Read the model definition and answer for the solid it produces. Units are mm, in the model's axes. A direction names the side the tool comes from. Coordinates: 2 decimals unless noted, no trailing zeros. Loops run counter-clockwise (first coordinate to the right, second up) from the corner with the lowest first, then second, coordinate; pieces in that order, holes last.
from build123d import *

# Parameters (mm, degrees)
SKETCH1_R           = 53.5
BOSS_EXTRUDE1_DEPTH = 2
SKETCH2_R           = 2.7
BOSS_EXTRUDE2_DEPTH = 2
SKETCH3_R           = 3.55
CUT_EXTRUDE1_DEPTH  = 2
SKETCH7_R           = 53.5
SKETCH7_R_2         = 52
BOSS_EXTRUDE3_DEPTH = 10
SKETCH8_W           = 56.651812746
SKETCH8_H           = 12.7
CUT_EXTRUDE4_DEPTH  = 10
SKETCH13_R          = 52.5
SKETCH13_R_2        = 3.55
BOSS_EXTRUDE4_DEPTH = 2
SKETCH12_R          = 2.75
CUT_EXTRUDE6_DEPTH  = 3
SKETCH16_R          = 1.5
CUT_EXTRUDE8_DEPTH  = 2


with BuildPart() as part:
    # Sketch1 → Boss-Extrude1 (new body)
    with BuildSketch(Plane(origin=(0, 0, 0), x_dir=(1, 0, 0), z_dir=(0, 1, 0))):
        Circle(SKETCH1_R)
    extrude(amount=BOSS_EXTRUDE1_DEPTH)

    # Sketch2 → Boss-Extrude2 (add)
    with BuildSketch(Plane(origin=(0, 2, 0), x_dir=(1, 0, 0), z_dir=(0, 1, 0))):
        with Locations((0, -44.45)):
            Circle(SKETCH2_R)
        with Locations((0, 44.45)):
            Circle(SKETCH2_R)
    extrude(amount=BOSS_EXTRUDE2_DEPTH)

    # Sketch3 → Cut-Extrude1 (cut)
    with BuildSketch(Plane(origin=(0, 2, 0), x_dir=(1, 0, 0), z_dir=(0, 1, 0))):
        Circle(SKETCH3_R)
    extrude(amount=-CUT_EXTRUDE1_DEPTH, mode=Mode.SUBTRACT)

    # Sketch7 → Boss-Extrude3 (add)
    with BuildSketch(Plane(origin=(0, 2, 0), x_dir=(1, 0, 0), z_dir=(0, 1, 0))):
        Circle(SKETCH7_R)
        Circle(SKETCH7_R_2, mode=Mode.SUBTRACT)
    extrude(amount=BOSS_EXTRUDE3_DEPTH)

    # Sketch8 → Cut-Extrude4 (cut)
    with BuildSketch(Plane(origin=(0, 2, 0), x_dir=(1, 0, 0), z_dir=(0, 1, 0))):
        with Locations((-28.325906373, 0)):
            Rectangle(SKETCH8_W, SKETCH8_H)
    extrude(amount=CUT_EXTRUDE4_DEPTH, mode=Mode.SUBTRACT)

    # Sketch13 → Boss-Extrude4 (add)
    with BuildSketch(Plane.XZ):
        Circle(SKETCH13_R)
        Circle(SKETCH13_R_2, mode=Mode.SUBTRACT)
    extrude(amount=BOSS_EXTRUDE4_DEPTH)

    # Sketch12 → Cut-Extrude6 (cut)
    with BuildSketch(Plane(origin=(0, 2, 0), x_dir=(1, 0, 0), z_dir=(0, 1, 0))):
        with Locations((11.16900504, 10.012658309)):
            Circle(SKETCH12_R)
        with Locations((-0.61610798, -14.987341691)):
            Circle(SKETCH12_R)
        with Locations((-13.568010506, 6.396021491)):
            Circle(SKETCH12_R)
    extrude(amount=-CUT_EXTRUDE6_DEPTH, mode=Mode.SUBTRACT)

    # Sketch16 → Cut-Extrude8 (cut, through all)
    with BuildSketch(Plane(origin=(0, -1, 0), x_dir=(1, 0, 0), z_dir=(0, 1, 0))):
        with Locations((11.16900504, 10.012658309)):
            Circle(SKETCH16_R)
        with Locations((-0.61610798, -14.987341691)):
            Circle(SKETCH16_R)
        with Locations((-13.568010506, 6.396021491)):
            Circle(SKETCH16_R)
    extrude(amount=-CUT_EXTRUDE8_DEPTH, mode=Mode.SUBTRACT)


solid = part.part
Q1. Flat-ended cylindrical pins translate along their axes: pin 1 Ø4.5 at (x, z) = (-1, -45.5) entering from +Y; pin 2 Ø9 at (x, z) = (-13.57, -6.4) entering from +Y; pin 3 Ø3.5 at (x, z) = (11.17, -10.01) entering from +Y; pin 4 Ø6.5 at (x, z) = (0, 0) entering from -Y. Find the tip coordinate at first contact, or state that the pin passes through.
Findings below:
pin 1: stops at y = 4
pin 2: stops at y = 2
pin 3: stops at y = -1
pin 4: passes through
Q2. Which of the six approach directions +Z, -Z, +X, -X, +Y, -Y give full straight-line access (tool end or side, diameter ignored) to faces 1 (the face through (35.4, 0, 39.4)), 2 (the face through (49.42, 5.92, 20.49)), 3 (the face through (1.246, 2.986, -42.055))?
Findings below:
face 1: -Y
face 2: +Y, -Y
face 3: +Y
Q3. Straight lines are drawn through the part: probe 1 along Y at (x, z) = (-44, -24); probe 2 along Z at (x, y) = (0, 1.25); probe 3 along Z at (x, y) = (19, 11.25). For each, find the intervals that lie inside material, in ascending order.
Findings below:
probe 1: y = -2 to 2
probe 2: z = -53.5 to -3.55, 3.55 to 12.31, 17.67 to 53.5
probe 3: z = -50.01 to -48.4, 48.4 to 50.01
Q4. A cutting plane is placed at A-A (z = 24). Give the vertices of the cut face in (x, y), then the cut area to 3 significant figures.
Findings below:
outline: (-47.81, 0) - (-46.69, 0) - (-46.69, -2) - (46.69, -2) - (46.69, 0) - (47.81, 0) - (47.81, 12) - (46.13, 12) - (46.13, 2) - (-46.13, 2) - (-46.13, 12) - (-47.81, 12) - close
area: 412 mm2
Q5. A cutting plane is placed at C-C (z = -44.45). Give the vertices of the cut face in (x, y), then the cut area to 3 significant figures.
Findings below:
outline: (-29.77, 0) - (-27.94, 0) - (-27.94, -2) - (27.94, -2) - (27.94, 0) - (29.77, 0) - (29.77, 12) - (26.99, 12) - (26.99, 2) - (2.7, 2) - (2.7, 4) - (-2.7, 4) - (-2.7, 2) - (-26.99, 2) - (-26.99, 12) - (-29.77, 12) - close
area: 297 mm2
Q6. Determine the mould class of faces 4 (the face through (9.67, -1.49, -10.08)), 5 (the face through (50.076, -0.986, 15.77)), 6 (the face through (-8, 12, -52)), 7 (the face through (0.77, -1.49, 15.56)) for opening direction Z: +Z half, -Z half, draft (parallel to the pull), parting line (faces both ways), or undercut.
Findings below:
face 4: undercut
face 5: parting line
face 6: draft
face 7: undercut
Q7. A cutting plane is placed at B-B (x = 18). Give the vertices of the cut face in (y, z).
Findings below:
outline: (-2, -49.32) - (0, -49.32) - (0, -50.38) - (12, -50.38) - (12, -48.79) - (2, -48.79) - (2, 48.79) - (12, 48.79) - (12, 50.38) - (0, 50.38) - (0, 49.32) - (-2, 49.32) - close
